from build123d import *

# Parameters (mm, degrees)
ESBO_O1_R                = 7.5
ESBO_O1_R_2              = 2
ESBO_O1_R_3              = 1.25
RESSALTO_EXTRUS_O1_DEPTH = 3
RESSALTO_EXTRUS_O2_START = 3
ESBO_O1_3_R              = 23.9
ESBO_O1_3_R_2            = 2
ESBO_O1_3_R_3            = 3.85
RESSALTO_EXTRUS_O2_DEPTH = 3
RESSALTO_EXTRUS_O3_START = 12
ESBO_O1_4_R              = 7.5
ESBO_O1_4_R_2            = 3.85
RESSALTO_EXTRUS_O3_DEPTH = 12
FILETE1_R                = 0.25
ESBO_O2_W                = 65
ESBO_O2_H                = 13.5
RESSALTO_EXTRUS_O4_DEPTH = 3
ESBO_O4_R                = 1.5
CORTE_EXTRUS_O1_DEPTH    = 3


with BuildPart() as part:
    # Esboço1 → Ressalto-extrusão1 (new body)
    with BuildSketch(Plane(origin=(0, 0, 0), x_dir=(1, 0, 0), z_dir=(0, 1, 0))):
        with BuildLine():
            Line((-39.65, 96.65), (25.35, 96.65))
            Line((25.35, 96.65), (25.35, 0))
            ThreePointArc((25.35, 0), (4.871403095, -24.877538702), (-23.477765829, -9.561224382))
            Line((-23.477765829, -9.561224382), (-38.911446086, 28.336467011))
            ThreePointArc((-38.911446086, 28.336467011), (-39.463624735, 30.186495131), (-39.65, 32.108153157))
            Line((-39.65, 32.108153157), (-39.65, 96.65))
        make_face()
        with Locations(Location((0, 0, 0), (0, 0, 270))):
            Circle(ESBO_O1_R, mode=Mode.SUBTRACT)
        with Locations(Location((0, 20, 0), (0, 0, 270))):
            Circle(ESBO_O1_R_2, mode=Mode.SUBTRACT)
        with Locations(Location((17.320508076, 10, 0), (0, 0, 270))):
            Circle(ESBO_O1_R_2, mode=Mode.SUBTRACT)
        with Locations(Location((17.320508076, -10, 0), (0, 0, 270))):
            Circle(ESBO_O1_R_2, mode=Mode.SUBTRACT)
        with Locations(Location((0, -20, 0), (0, 0, 270))):
            Circle(ESBO_O1_R_2, mode=Mode.SUBTRACT)
        with Locations(Location((-17.320508076, -10, 0), (0, 0, 270))):
            Circle(ESBO_O1_R_2, mode=Mode.SUBTRACT)
        with Locations(Location((-17.320508076, 10, 0), (0, 0, 270))):
            Circle(ESBO_O1_R_2, mode=Mode.SUBTRACT)
        with Locations(Location((20.35, 92.65, 0), (0, 0, 270))):
            Circle(ESBO_O1_R_3, mode=Mode.SUBTRACT)
        with Locations(Location((-1.65, 92.65, 0), (0, 0, 270))):
            Circle(ESBO_O1_R_3, mode=Mode.SUBTRACT)
        with Locations(Location((-25.65, 92.65, 0), (0, 0, 270))):
            Circle(ESBO_O1_R_3, mode=Mode.SUBTRACT)
    extrude(amount=-RESSALTO_EXTRUS_O1_DEPTH)

    # Esboço1<3> → Ressalto-extrusão2 (add)
    with BuildSketch(Plane(origin=(0, 0, 0), x_dir=(1, 0, 0), z_dir=(0, 1, 0)).offset(RESSALTO_EXTRUS_O2_START)):
        with Locations(Location((0, 0, 0), (0, 0, 270))):
            Circle(ESBO_O1_3_R)
        with Locations(Location((-17.320508076, -10, 0), (0, 0, 270))):
            Circle(ESBO_O1_3_R_2, mode=Mode.SUBTRACT)
        with Locations(Location((-17.320508076, 10, 0), (0, 0, 270))):
            Circle(ESBO_O1_3_R_2, mode=Mode.SUBTRACT)
        with Locations(Location((0, -20, 0), (0, 0, 270))):
            Circle(ESBO_O1_3_R_2, mode=Mode.SUBTRACT)
        with Locations(Location((17.320508076, -10, 0), (0, 0, 270))):
            Circle(ESBO_O1_3_R_2, mode=Mode.SUBTRACT)
        with Locations(Location((0, 20, 0), (0, 0, 270))):
            Circle(ESBO_O1_3_R_2, mode=Mode.SUBTRACT)
        with Locations(Location((17.320508076, 10, 0), (0, 0, 270))):
            Circle(ESBO_O1_3_R_2, mode=Mode.SUBTRACT)
        with Locations(Location((0, 0, 0), (0, 0, 270))):
            Circle(ESBO_O1_3_R_3, mode=Mode.SUBTRACT)
    extrude(amount=-RESSALTO_EXTRUS_O2_DEPTH)

    # Esboço1<4> → Ressalto-extrusão3 (add)
    with BuildSketch(Plane(origin=(0, 0, 0), x_dir=(1, 0, 0), z_dir=(0, 1, 0)).offset(RESSALTO_EXTRUS_O3_START)):
        with Locations(Location((0, 0, 0), (0, 0, 270))):
            Circle(ESBO_O1_4_R)
        with Locations(Location((0, 0, 0), (0, 0, 270))):
            Circle(ESBO_O1_4_R_2, mode=Mode.SUBTRACT)
    extrude(amount=-RESSALTO_EXTRUS_O3_DEPTH)

    # Filete1
    filete1_edges = [part.edges().sort_by_distance(p)[0] for p in [
        (0, 12, -3.85),
        (0, 12, -7.5),
    ]]
    fillet(filete1_edges, radius=FILETE1_R)

    # Esboço2 → Ressalto-extrusão4 (add)
    with BuildSketch(Plane(origin=(0, 0, -96.65), x_dir=(-1, 0, 0), z_dir=(0, 0, -1))):
        with Locations((7.15, 3.75)):
            Rectangle(ESBO_O2_W, ESBO_O2_H)
    extrude(amount=RESSALTO_EXTRUS_O4_DEPTH)

    # Esboço4 → Corte-extrusão1 (cut)
    with BuildSketch(Plane(origin=(0, 0, -99.65), x_dir=(-1, 0, 0), z_dir=(0, 0, -1))):
        with Locations((-11.35, 5.5)):
            Circle(ESBO_O4_R)
        with Locations((13.65, 5.5)):
            Circle(ESBO_O4_R)
        with Locations((38.65, 5.5)):
            Circle(ESBO_O4_R)
    extrude(amount=-CORTE_EXTRUS_O1_DEPTH, mode=Mode.SUBTRACT)


solid = part.part
Check sheet for the modelled part. Datum: model origin and axes. Units: mm. A direction names the side the tool comes from. Round coordinates to 2 decimals unless told otherwise and drop trailing zeros. Order: outer loops, then holes, each group sorted by start corner. A loop starts at its lowest first (then second) coordinate and runs counter-clockwise, first axis right, second up.
(1) Cross-section at B-B, the plane x = -25.65. Enter the section's corners in (y, z).
(2) Access from +Z, -Z, +X, -X, +Y, -Y to the whole of each face (thin tool, end or side, straight path). Record for faces 4 (the cylindrical face through (-39.46, -1.48, -30.16)), 5 (the flat face through (-7, 5, -96.65)), 6 (the flat face through (-3, 0, 3)).
(3) Draft check along Z on faces 1 (the cylindrical face through (-1.2, 0, 18.4)), 2 (the cylindrical face through (-12.15, 5.57, -98.17)), 3 (the cylindrical face through (5.35, -1.48, 24.78)). Enter one of: pulls with the +Z half, pulls with the -Z half, needs draft (parallel to the pull), parting line crosses it, or undercut.
(4) Cross-section at C-C, the plane z = -20. Enter the section's corners in (x, y).
(5) Cross-section at D-D, the plane x = 11.35. Enter the section's corners in (y, z).
(6) Cross-section at A-A, the plane z = -92.65. Enter the section's corners in (x, y).
(7) Go/stop test with flat-tipped pins: P1, Ø4, axis at x = -25.65, z = -92.65, coming from the +Y side; P2, Ø1.5, axis at x = -6.5, z = -11.5, coming from the +Y side; P3, Ø2, axis at y = 2.5, z = -45, coming from the -X side (1 decimal); P4, Ø2.5, axis at x = -19.5, z = -98, coming from the +Y side. Record where each tip stops, or that it passes through.
(8) Scan lines: probe 1 along X at (y, z) = (-1.7, -92.65); probe 2 along X at (y, z) = (2.5, -11.5); probe 3 along Z at (x, y) = (2.5, 1.5). Record each from-to range of solid material in increasing order.
Check sheet entries:
1. outline: (-3, -99.65) - (10.5, -99.65) - (10.5, -96.65) - (0, -96.65) - (0, -93.9) - (-3, -93.9) - close; (-3, -91.4) - (0, -91.4) - (0, 4.23) - (-3, 4.23) - close
2. face 4: +Z, -X, +Y, -Y
2. face 5: +X, -X, +Y
2. face 6: -Y
3. face 1: undercut
3. face 2: needs draft
3. face 3: pulls with the +Z half
4. outline: (-35.52, -3) - (-2, -3) - (-2, 3) - (-13.08, 3) - (-13.08, 0) - (-35.52, 0) - close; (2, -3) - (25.35, -3) - (25.35, 0) - (13.08, 0) - (13.08, 3) - (2, 3) - close
5. outline: (-3, -99.65) - (4, -99.65) - (4, -96.65) - (0, -96.65) - (0, -21.03) - (3, -21.03) - (3, 21.03) - (0, 21.03) - (0, 22.67) - (-3, 22.67) - close; (7, -99.65) - (10.5, -99.65) - (10.5, -96.65) - (7, -96.65) - close
6. outline: (-39.65, -3) - (-26.9, -3) - (-26.9, 0) - (-39.65, 0) - close; (-24.4, -3) - (-2.9, -3) - (-2.9, 0) - (-24.4, 0) - close; (-0.4, -3) - (19.1, -3) - (19.1, 0) - (-0.4, 0) - close; (21.6, -3) - (25.35, -3) - (25.35, 0) - (21.6, 0) - close
7. P1: stops at y = 0
7. P2: stops at y = 3
7. P3: passes through
7. P4: stops at y = 10.5
8. probe 1: x = -39.65 to -26.9, -24.4 to -2.9, -0.4 to 19.1, 21.6 to 25.35
8. probe 2: x = -20.95 to -18.64, -16 to 16, 18.64 to 20.95
8. probe 3: z = -99.65 to -96.65, -23.77 to -2.93, 2.93 to 23.77
